The listing builds one solid part. Answer for the finished solid, in the listing's coordinates (mm). Face numbers are marked on the shaded views. A direction names the side the tool comes from. Coordinates: 2 decimals unless noted, no trailing zeros. Order: outer loops, then holes, each group sorted by start corner. A loop starts at its lowest first (then second) coordinate and runs counter-clockwise, first axis right, second up. Notation, with made-up numbers: (1.25, 36) -> (19.25, 36) arc R26 cw to (19.25, 50) -> close; hole circle Ø2 at (13, -3.75). An arc over 180 degrees is marked (long way). Return JSON: item names as keys, results as strings.
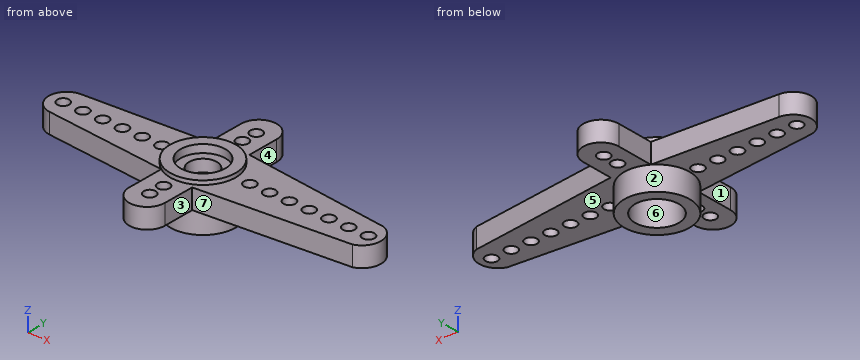
Solid Edge part; units mm, degrees
sketch "Sketch1" plane through (0, 0, 0) normal (0, 0, 1) x (1, 0, 0)
  circle A0 centre (0, 0) radius 3.3
extrude "Protrusion1" add sketch "Sketch1" along normal blind 4.8
sketch "Sketch2" plane through (0, 0, 4.8) normal (0, 0, 1) x (1, 0, 0)
  circle A0 centre (0, 0) radius 2.25
extrude "Extrusionsausschnitt_1" cut sketch "Sketch2" against normal blind 0.8
sketch "Sketch3" plane through (0, 0, 4) normal (0, 0, 1) x (1, 0, 0)
  circle A0 centre (0, 0) radius 1.4
extrude "Cutout1" cut sketch "Sketch3" against normal through all
sketch "Sketch4" plane through (0, 0, 0) normal (0, 0, -1) x (1, 0, 0)
  circle A0 centre (0, 0) radius 2.2
extrude "Extrusionsausschnitt_3" cut sketch "Sketch4" against normal blind 2.8
sketch "Sketch5" plane through (0, 0, 2.4) normal (0, 0, -1) x (1, 0, 0)
  line L0 (-13.9375, 1.8) -> (-1.8, 2.7659)
  line L1 (-1.8, 2.7659) -> (-1.8, 6.45)
  arc A0 (-1.8, 6.45) -> (1.8, 6.45) centre (0, 6.45) cw
  line L2 (1.8, 6.45) -> (1.8, 3.3)
  line L3 (1.8, 3.3) -> (16.7, 1.8)
  arc A1 (16.7, 1.8) -> (16.7, -1.8) centre (16.1038, 0) cw
  line L4 (1.8, -3.3) -> (16.7, -1.8)
  line L5 (1.8, -6.45) -> (1.8, -3.3)
  arc A2 (-1.8, -6.45) -> (1.8, -6.45) centre (0, -6.45) ccw
  line L6 (-1.8, -2.7659) -> (-1.8, -6.45)
  line L7 (-13.9375, -1.8) -> (-1.8, -2.7659)
  arc A3 (-13.9375, 1.8) -> (-13.9375, -1.8) centre (-13.7943, 0) ccw
  circle A4 centre (0, 0) radius 2.7122
extrude "Extrusionsausprägung_2" add sketch "Sketch5" against normal blind 2
sketch "Sketch6" plane through (0, 0, 0) normal (0, 0, 1) x (1, 0, 0)
  circle A0 centre (0, 6.15) radius 0.6
  circle A1 centre (0, 4.55) radius 0.6
extrude "Cutout2" cut sketch "Sketch6" along normal through all
mirror "Mirror1" about plane through (0, 0, 0) normal (0, -1, 0) of "Cutout2"
sketch "Sketch7" plane through (0, 0, 0) normal (0, 0, 1) x (1, 0, 0)
  circle A0 centre (-12.15, 0) radius 0.6
  circle A1 centre (-14.15, 0) radius 0.6
  circle A2 centre (-10.15, 0) radius 0.6
  circle A3 centre (-8.15, 0) radius 0.6
  circle A4 centre (-6.15, 0) radius 0.6
  circle A5 centre (-4.15, 0) radius 0.6
  dimension "D1" = 12.15
extrude "Cutout3" cut sketch "Sketch7" along normal through all
sketch "Sketch8" plane through (0, 0, 0) normal (0, 0, 1) x (1, 0, 0)
  circle A0 centre (4.75, 0) radius 0.6
  circle A1 centre (6.75, 0) radius 0.6
  circle A2 centre (8.75, 0) radius 0.6
  circle A3 centre (10.75, 0) radius 0.6
  circle A4 centre (12.75, 0) radius 0.6
  circle A5 centre (14.75, 0) radius 0.6
  circle A6 centre (16.75, 0) radius 0.6
extrude "Cutout4" cut sketch "Sketch8" along normal through all
Item 1: The part is cut by section C-C on y = 0. Count the separate pieces of the cut face and the enclosed holes in it, plus the area to 3 significant figures.
Answer list:
{"separate pieces": "15", "enclosed holes": "0", "area": "35.2 mm2"}
Item 2: Determine the mould class of the marked faces 5, 6 and 7 for opening direction Y: pulls with the +Y half, pulls with the -Y half, needs draft (parallel to the pull), parting line crosses it, or undercut.
Answer list:
{"face 5": "needs draft", "face 6": "undercut", "face 7": "pulls with the -Y half"}
Item 3: Flat-ended cylindrical pins translate along their axes: pin 1 (0.7 mm diameter, centred on x = -10.15, y = 0, fed in from -Z); pin 2 (1.6 mm diameter, centred on y = 5, z = 3.5, fed in from +X); pin 3 (1.9 mm diameter, centred on x = 0, y = 4.55, fed in from +Z); pin 4 (2 mm diameter, centred on x = 14, z = 2.5, fed in from -Y). Find the tip coordinate at first contact, or state that the pin passes through.
Answer list:
{"pin 1": "through", "pin 2": "x = 1.8", "pin 3": "z = 4.4", "pin 4": "y = -2.17"}
Item 4: Which of the six approach directions +Z, -Z, +X, -X, +Y, -Y give full straight-line access (tool end or side, diameter ignored) to the marked faces 1, 2, 3 and 4?
Answer list:
{"face 1": "+Z, -Z, -X, -Y", "face 2": "-Z", "face 3": "+Z, -Z, +X, -Y", "face 4": "+Z, -Z, +X, +Y"}
Item 5: The part is cut by section A-A on x = -6.15. Determine the outline of the cut face in (y, z).
Answer list:
{"outline": "(-2.42, 2.4) -> (-0.6, 2.4) -> (-0.6, 4.4) -> (-2.42, 4.4) -> close; (0.6, 2.4) -> (2.42, 2.4) -> (2.42, 4.4) -> (0.6, 4.4) -> close"}
Item 6: The part is cut by section D-D on x = 6.75. Determine the outline of the cut face in (y, z), plus the area to 3 significant figures.
Answer list:
{"outline": "(-2.8, 2.4) -> (-0.6, 2.4) -> (-0.6, 4.4) -> (-2.8, 4.4) -> close; (0.6, 2.4) -> (2.8, 2.4) -> (2.8, 4.4) -> (0.6, 4.4) -> close", "area": "8.81 mm2"}
Item 7: The part is cut by section B-B on z = 0.55. Determine the outline of the cut face in (x, y), plus the area to 3 significant figures.
Answer list:
{"outline": "circle Ø6.6 at (0, 0); hole circle Ø4.4 at (0, 0)", "area": "19.0 mm2"}
Item 8: Find the intervals of material crossed by probe 1 along Y at (x, z) = (0, 3.5); probe 2 along X at (y, z) = (0, 1.65), in increasing order.
Answer list:
{"probe 1": "-8.25 to -6.75, -5.55 to -5.15, -3.95 to -1.4, 1.4 to 3.95, 5.15 to 5.55, 6.75 to 8.25", "probe 2": "-3.3 to -2.2, 2.2 to 3.3"}
